Read the model definition and answer for the solid it produces. Units are mm, in the model's axes. Face numbers are marked on the shaded views. Coordinates: 2 decimals unless noted, no trailing zeros. Write each loop counter-clockwise with the first axis right and the second up, starting at its lowest first coordinate (ties: lowest second). Pieces come first, ordered by that corner, then holes.
(1) The part is cut by section A-A, the plane y = 352.3. Determine the outline of the cut face in (x, z).
(2) Determine the mould class of the marked faces 1, 2 and 3 for opening direction X: pulls with the +X half, pulls with the -X half, needs draft (parallel to the pull), parting line crosses it, or undercut.
(3) The part is cut by section D-D, the plane y = 375. Determine the outline of the cut face in (x, z), and give its area (3 significant figures).
(4) Given pin 1 (6 mm diameter, centred on x = -290, z = 655.5, fed in from -Y); pin 2 (1 mm diameter, centred on x = -300, z = 666.5, fed in from -Y); pin 3 (2 mm diameter, centred on x = -304, z = 644.5, fed in from -Y), each flat-ended and moving along its own axis, determine where each tip first touches the part or whether it passes through.
(5) Straight lines are drawn through the part: line 1 along X through (y, z) = (352, 635); line 2 along Y through (x, z) = (-299, 648); line 3 along X through (y, z) = (361.5, 654). For each, find the intervals that lie inside material, in ascending order.
(6) The part is cut by section B-B, the plane x = -300. Determine the outline of the cut face in (y, z).
(7) The part is cut by section C-C, the plane z = 636.5. Determine the outline of the cut face in (x, y).
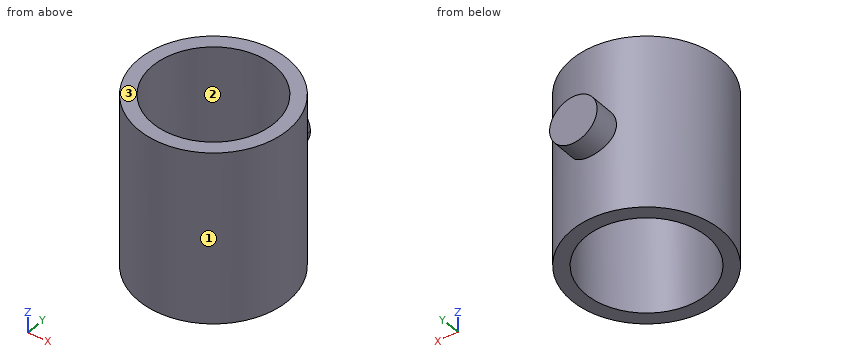
```python
from build123d import *

# Parameters (mm, degrees)
SKETCH1_R                = 21.5
BOSS_EXTRUDE1_DEPTH      = 50
SKETCH2_R                = 17.5
CUT_EXTRUDE1_DEPTH       = 495.985656358
BOSS_EXTRUDE2_REACH      = 750.708
BOSS_EXTRUDE2_END_RADIUS = 21.5


with BuildPart() as part:
    # Sketch1 → Boss-Extrude1 (new body)
    with BuildSketch(Plane(origin=(0, 0, 624.8), x_dir=(-1, 0, 0), z_dir=(0, 0, -1))):
        with Locations(Location((299.1, 352.3, 0), (0, 0, 180))):
            Circle(SKETCH1_R)
    extrude(amount=-BOSS_EXTRUDE1_DEPTH)

    # Sketch2 → Cut-Extrude1 (cut, through all)
    with BuildSketch(Plane.XY.offset(674.8)):
        with Locations(Location((-299.1, 352.3, 0), (0, 0, 180))):
            Circle(SKETCH2_R)
    extrude(amount=-CUT_EXTRUDE1_DEPTH, mode=Mode.SUBTRACT)

    # Boss-Extrude2: up to this cylinder (the profile starts outside it)
    boss_extrude2_end = Plane(origin=(-299.1, 352.3, 649.8), z_dir=(0, 0, -1)) * Cylinder(BOSS_EXTRUDE2_END_RADIUS, 1545.416, mode=Mode.PRIVATE)
    # Sketch3 → Boss-Extrude2 (add, up to the surface)
    with BuildSketch(Plane(origin=(0, 380.036620923, 0), x_dir=(1, 0, 0), z_dir=(0, 1, 0)), mode=Mode.PRIVATE) as boss_extrude2_sk1:
        with BuildLine():
            ThreePointArc((-292.280237329, -649.8), (-294.277699569, -654.622300431), (-299.1, -656.619762671))
            ThreePointArc((-299.1, -656.619762671), (-303.922300431, -644.977699569), (-292.280237329, -649.8))
        make_face()
    boss_extrude2_tool1 = extrude(boss_extrude2_sk1.sketch, amount=-BOSS_EXTRUDE2_REACH, mode=Mode.PRIVATE) - boss_extrude2_end
    add(boss_extrude2_tool1.solids().sort_by_distance((-299.1, 380.036621, 649.8))[0])


solid = part.part
```
Computed:
1. outline: (-320.6, 624.8) - (-316.6, 624.8) - (-316.6, 674.8) - (-320.6, 674.8) - close; (-281.6, 624.8) - (-277.6, 624.8) - (-277.6, 674.8) - (-281.6, 674.8) - close
2. face 1: parting line crosses it
2. face 2: undercut
2. face 3: needs draft
3. outline: circle Ø13.64 at (-299.1, 649.8)
3. area: 146 mm2
4. pin 1: stops at y = 331.68
4. pin 2: stops at y = 330.8
4. pin 3: stops at y = 331.16
5. line 1: x = -320.6 to -316.6, -281.6 to -277.6
5. line 2: y = 330.8 to 334.8, 369.8 to 380.04
5. line 3: x = -318.53 to -313.99, -284.21 to -279.67
6. outline: (330.82, 624.8) - (334.82, 624.8) - (334.82, 674.8) - (330.82, 674.8) - close; (369.78, 624.8) - (373.78, 624.8) - (373.78, 643.04) - (380.04, 643.04) - (380.04, 656.56) - (373.78, 656.56) - (373.78, 674.8) - (369.78, 674.8) - close
7. outline: circle Ø43 at (-299.1, 352.3); hole circle Ø35 at (-299.1, 352.3)
